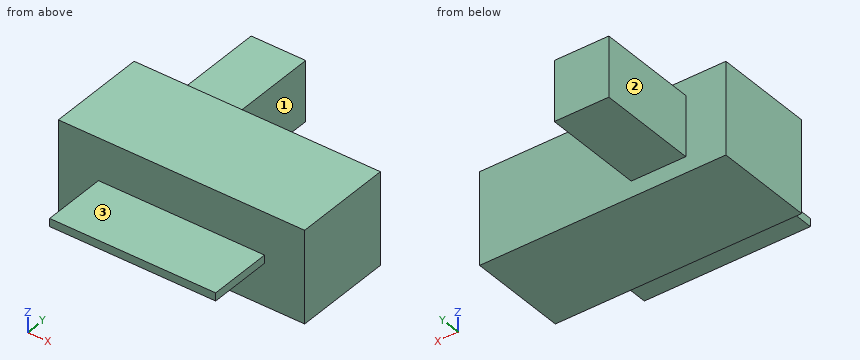
```python
from build123d import *

# Parameters (mm, degrees)
ESBO_O2_W                = 15.35
ESBO_O2_H                = 5.75
ESBO_O2_W_2              = 10.35
ESBO_O2_H_2              = 3.75
ESBO_O2_W_3              = 3.4
ESBO_O2_W_4              = 6.95
RESSALTO_EXTRUS_O1_DEPTH = 6.2
ESBO_O2_3_W              = 3.4
ESBO_O2_3_H              = 3.75
RESSALTO_EXTRUS_O2_DEPTH = 6.3
RESSALTO_EXTRUS_O3_DEPTH = 4


with BuildPart() as part:
    # Esbo_o2 → Ressalto-extrus_o1 (new body)
    # profile 1 of 3: a face of its own
    with BuildSketch(Plane(origin=(0, 0, 0), x_dir=(1, 0, 0), z_dir=(0, 1, 0))):
        with Locations((7.675, 2.875)):
            Rectangle(ESBO_O2_W, ESBO_O2_H)
        with Locations((7.675, 2.875)):
            Rectangle(ESBO_O2_W_2, ESBO_O2_H_2, mode=Mode.SUBTRACT)
    # profile 2 of 3: a face of its own
    with BuildSketch(Plane(origin=(0, 0, 0), x_dir=(1, 0, 0), z_dir=(0, 1, 0))):
        with Locations((4.2, 2.875)):
            Rectangle(ESBO_O2_W_3, ESBO_O2_H_2)
    # profile 3 of 3: a face of its own
    with BuildSketch(Plane(origin=(0, 0, 0), x_dir=(1, 0, 0), z_dir=(0, 1, 0))):
        with Locations((9.375, 2.875)):
            Rectangle(ESBO_O2_W_4, ESBO_O2_H_2)
    extrude(amount=-RESSALTO_EXTRUS_O1_DEPTH)

    # Esbo_o2_3 → Ressalto-extrus_o2 (add)
    with BuildSketch(Plane(origin=(0, 0, 0), x_dir=(1, 0, 0), z_dir=(0, 1, 0))):
        with Locations((4.2, 2.875)):
            Rectangle(ESBO_O2_3_W, ESBO_O2_3_H)
    extrude(amount=RESSALTO_EXTRUS_O2_DEPTH)

    # Esbo_o3 → Ressalto-extrus_o3 (add)
    with BuildSketch(Plane.XZ.offset(6.2)):
        Polygon((2.5, -2.875), (2.5, -2.625), (12.85, -2.625), (12.85, -2.875), (12.85, -3.125), (2.5, -3.125), align=None)
    extrude(amount=RESSALTO_EXTRUS_O3_DEPTH)


solid = part.part
```
The listing builds one solid part. Answer for the finished solid, in the listing's coordinates (mm). Face numbers are marked on the shaded views. A direction names the side the tool comes from. Coordinates: 2 decimals unless noted, no trailing zeros. Loops run counter-clockwise (first coordinate to the right, second up) from the corner with the lowest first, then second, coordinate; pieces in that order, holes last. Notation, with made-up numbers: M 58,-23.5 L 110,-23.5 A11 ccw 110,-7.5 Z; hole C -3,51.25 d8. An arc over 180 degrees is marked long. Answer as CSV lines item,"result". Start each with the question number.
(1) The part is cut by section C-C (y = -8). Give the vertices of the cut face in (x, z) (3 decimals).
(2) The part is cut by section D-D (x = 11.5). Give the vertices of the cut face in (y, z) (3 decimals), and give its area (4 significant figures).
(3) Find the intervals of material crossed by L1, parallel to Y at x = 12, z = -0.35; L2, parallel to Y at x = 3.75, z = -4.4; L3, parallel to X at y = 3, z = -3, in increasing order. Write a range as [from, to].
(4) Given pin 1 (1 mm diameter, centred on x = 3.5, y = 2, fed in from +Z); pin 2 (1 mm diameter, centred on y = 1.5, z = -1.5, fed in from +X); pin 3 (1.2 mm diameter, centred on x = 8, y = -7.5, fed in from -Z) (3 decimals), each flat-ended and moving along its own axis, determine where each tip first touches the part or whether it passes through.
(5) For the marked faces 1, 2 and 3, determine the directions among +Z, -Z, +X, -X, +Y, -Y from which every point of the face is accessible in a straight line to the end or side of a thin tool.
(6) The part is cut by section A-A (x = 2.75). Give the vertices of the cut face in (y, z) (3 decimals), and give its area (3 significant figures).
(7) The part is cut by section B-B (z = -3.55). Give the vertices of the cut face in (x, y), and give its area (3 significant figures).
Determined:
1,outline,"M 2.5,-3.125 L 12.85,-3.125 L 12.85,-2.625 L 2.5,-2.625 Z"
2,outline,"M -10.2,-3.125 L -6.2,-3.125 L -6.2,-5.75 L 0,-5.75 L 0,0 L -6.2,0 L -6.2,-2.625 L -10.2,-2.625 Z"
2,area,"37.65 mm2"
3,L1,"[-6.2, 0]"
3,L2,"[-6.2, 6.3]"
3,L3,"[2.5, 5.9]"
4,pin 1,"z = -1"
4,pin 2,"x = 5.9"
4,pin 3,"z = -3.125"
5,face 1,"+Z, -Z, +X, +Y"
5,face 2,"+Z, -Z, -X, +Y"
5,face 3,"+Z, +X, -X, -Y"
6,outline,"M -10.2,-3.125 L -6.2,-3.125 L -6.2,-5.75 L 0,-5.75 L 0,-4.75 L 6.3,-4.75 L 6.3,-1 L 0,-1 L 0,0 L -6.2,0 L -6.2,-2.625 L -10.2,-2.625 Z"
6,area,"61.3 mm2"
7,outline,"M 0,-6.2 L 15.35,-6.2 L 15.35,0 L 5.9,0 L 5.9,6.3 L 2.5,6.3 L 2.5,0 L 0,0 Z"
7,area,"117 mm2"
